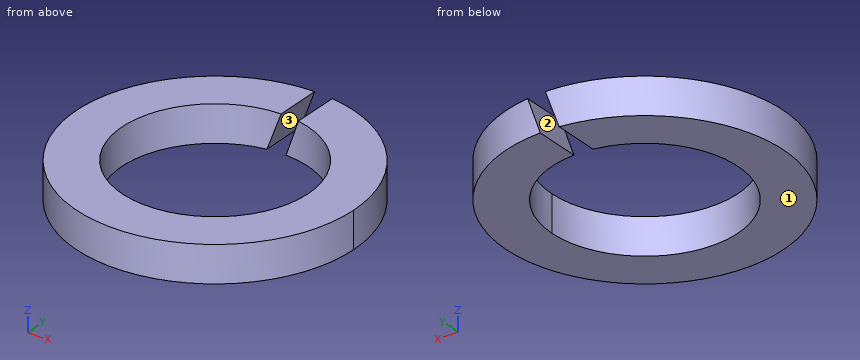
Autodesk Inventor part; units mm, degrees
ref_plane "Work Plane1" through (0, 0, 0) normal (1, 0, 0) x (0, 1, 0)
ref_plane "XZ Plane" through (0, 0, 0) normal (0, 1, 0) x (-1, 0, 0)
ref_plane "XY Plane" through (0, 0, 0) normal (0, 0, 1) x (1, 0, 0)
sketch "Sketch1" plane through (0, 0, 0) normal (0, 0, 1) x (1, 0, 0)
  circle A0 centre (0, 0) radius 7.6
  circle A1 centre (0, 0) radius 5.1
  line L0 (-2.59, 0) -> (2.59, 0) construction
  line L1 (0, -2.59) -> (0, 2.59) construction
  dimension "d0" = 15.2
  dimension "d1" = 10.2
extrude "Выдавливание1" add sketch "Sketch1" along normal blind 2
sketch "Sketch2" plane through (0, 0, 0) normal (0, 1, 0) x (-1, 0, 0)
  line L0 (-5.1, 2) -> (5.1, 2) construction
  line L1 (5.1, 0) -> (-5.1, 0) construction
  line L2 (-0.864, 2) -> (-0.136, 0)
  line L3 (0.136, 2) -> (0.864, 0)
  line L4 (0, 0) -> (0, 2) construction
  line L5 (0, 1) -> (-0.364, 2) construction
  line L6 (-0.864, 2) -> (0.136, 2)
  line L7 (-0.136, 0) -> (0.864, 0)
  dimension "d4" = 70
  dimension "d13" = 1
extrude "Выдавливание2" cut sketch "Sketch2" along normal through all
ref_plane "Work Plane1" through (0, 0, 0) normal (1, 0, 0) x (0, 1, 0)
equation "\"d0\" = d + 2 * b"
equation "\"d1\" = d"
equation "\"d2\" = s_"
equation "\"d4\" = Angle"
equation "\"d13\" = 0.5 * s_"
equation "\"d7\" = s_"
equation "\"d\" = 10.2"
equation "\"b\" = 2.5"
equation "\"s_\" = 2"
equation "\"D_\" = 15.2"
equation "\"Angle\" = 70deg"
properties part number "Шайба 2 10Л ГОСТ 6402-78" material "Сталь, мягкая"
The listing builds one solid part. Answer for the finished solid, in the listing's coordinates (mm). Face numbers are marked on the shaded views. Give positions to 0.01 mm unless a question says otherwise; leave off trailing zeros. Write each loop counter-clockwise with the first axis right and the second up, starting at its lowest first coordinate (ties: lowest second). Pieces come first, ordered by that corner, then holes. Notation, with made-up numbers: (23.25, -28) -> (71.25, -28) arc R23 cw to (71.25, 7) -> close; hole circle Ø5 at (19, 81.5). An arc over 180 degrees is marked (long way). Use one line per item in the form item = value.
1) Section C-C on z = 1 is taken. Write down the section's boundary in (x, y), plus the area to 3 significant figures.
Result:
outline = (-0.5, 5.08) -> (-0.5, 7.58) arc R7.6 ccw (long way) to (0.5, 7.58) -> (0.5, 5.08) arc R5.1 cw (long way) to start
area = 97.2 mm²
2) For a pull along X with two mould halves and no side action, classify the marked faces 1, 2 and 3 as +X half, -X half, draft (parallel to the pull), parting line (faces both ways), or undercut.
Result:
face_1 = draft
face_2 = undercut
face_3 = undercut
3) Section B-B on y = -1.25 is taken. Write down the section's boundary in (x, z).
Result:
outline = (-7.5, 0) -> (-4.94, 0) -> (-4.94, 2) -> (-7.5, 2) -> close; (4.94, 0) -> (7.5, 0) -> (7.5, 2) -> (4.94, 2) -> close
4) This flat-tipped pin is pushed along its axis until it touches: P1, Ø1.5, axis at x = 2.5, y = -6, coming from the -Z side. Where does it stop, or does it pass through?
Result:
P1 = 0
5) Straight lines are drawn through the part: probe 1 along X at (y, z) = (0, 1.15); probe 2 along X at (y, z) = (2.5, 0.9); probe 3 along Y at (x, z) = (0, 0.2). For each, find the intervals that lie inside material, in ascending order.
Result:
probe_1 = -7.6 to -5.1, 5.1 to 7.6
probe_2 = -7.18 to -4.45, 4.45 to 7.18
probe_3 = -7.6 to -5.1
6) Section A-A on x = -3.5 is taken. Write down the section's boundary in (y, z), plus the area to 3 significant figures.
Result:
outline = (-6.75, 0) -> (-3.71, 0) -> (-3.71, 2) -> (-6.75, 2) -> close; (3.71, 0) -> (6.75, 0) -> (6.75, 2) -> (3.71, 2) -> close
area = 12.1 mm²
